```python
from build123d import *

# Parameters (mm, degrees)
SKETCH_1_R      = 1.55
SKETCH_1_R_2    = 14
EXTRUDE_1_DEPTH = 2


with BuildPart() as part:
    # 草图1 → 凸台-拉伸1 (new body)
    with BuildSketch(Plane.XY):
        Polygon((-90.5, 18), (-90.5, -18), (-62.5, -18), (-62.5, -46), (62.5, -46), (62.5, -18), (90.5, -18), (90.5, 18), (62.5, 18), (62.5, 46), (-62.5, 46), (-62.5, 18), align=None)
        with Locations((-52.935028843, -13.435028843)):
            Circle(SKETCH_1_R, mode=Mode.SUBTRACT)
        with Locations((-52.935028843, 13.435028843)):
            Circle(SKETCH_1_R, mode=Mode.SUBTRACT)
        with Locations((-26.064971157, -13.435028843)):
            Circle(SKETCH_1_R, mode=Mode.SUBTRACT)
        with Locations((-26.064971157, 13.435028843)):
            Circle(SKETCH_1_R, mode=Mode.SUBTRACT)
        with Locations((-39.5, 0)):
            Circle(SKETCH_1_R_2, mode=Mode.SUBTRACT)
        with Locations((39.5, 0)):
            Circle(SKETCH_1_R_2, mode=Mode.SUBTRACT)
        with Locations((57.5, -43)):
            Circle(SKETCH_1_R, mode=Mode.SUBTRACT)
        with Locations((37.5, -43)):
            Circle(SKETCH_1_R, mode=Mode.SUBTRACT)
        with Locations((-57.5, -43)):
            Circle(SKETCH_1_R, mode=Mode.SUBTRACT)
        with Locations((-37.5, -43)):
            Circle(SKETCH_1_R, mode=Mode.SUBTRACT)
        with Locations((-57.5, 43)):
            Circle(SKETCH_1_R, mode=Mode.SUBTRACT)
        with Locations((-37.5, 43)):
            Circle(SKETCH_1_R, mode=Mode.SUBTRACT)
        with Locations((37.5, 43)):
            Circle(SKETCH_1_R, mode=Mode.SUBTRACT)
        with Locations((57.5, 43)):
            Circle(SKETCH_1_R, mode=Mode.SUBTRACT)
        with Locations((15, -43)):
            Circle(SKETCH_1_R, mode=Mode.SUBTRACT)
        with Locations((-5, -43)):
            Circle(SKETCH_1_R, mode=Mode.SUBTRACT)
        with Locations((-5, 43)):
            Circle(SKETCH_1_R, mode=Mode.SUBTRACT)
        with Locations((15, 43)):
            Circle(SKETCH_1_R, mode=Mode.SUBTRACT)
        with Locations((-87.5, 8)):
            Circle(SKETCH_1_R, mode=Mode.SUBTRACT)
        with Locations((-87.5, -2)):
            Circle(SKETCH_1_R, mode=Mode.SUBTRACT)
        with Locations((87.5, 8)):
            Circle(SKETCH_1_R, mode=Mode.SUBTRACT)
        with Locations((87.5, -2)):
            Circle(SKETCH_1_R, mode=Mode.SUBTRACT)
        with Locations((26.064971157, 13.435028843)):
            Circle(SKETCH_1_R, mode=Mode.SUBTRACT)
        with Locations((52.935028843, 13.435028843)):
            Circle(SKETCH_1_R, mode=Mode.SUBTRACT)
        with Locations((52.935028843, -13.435028843)):
            Circle(SKETCH_1_R, mode=Mode.SUBTRACT)
        with Locations((26.064971157, -13.435028843)):
            Circle(SKETCH_1_R, mode=Mode.SUBTRACT)
        with BuildLine():
            Line((-81.106273476, 14), (-65, 14))
            ThreePointArc((-65, 14), (-64.646446609, 13.853553391), (-64.5, 13.5))
            Line((-64.5, 13.5), (-64.5, -10.235560912))
            ThreePointArc((-64.5, -10.235560912), (-64.853147938, -10.713509101), (-65.413737887, -10.516311621))
            Line((-65.413737887, -10.516311621), (-81.520011363, 13.219249291))
            ThreePointArc((-81.520011363, 13.219249291), (-81.548073971, 13.734120317), (-81.106273476, 14))
        make_face(mode=Mode.SUBTRACT)
        with BuildLine():
            Line((-66.893726524, -14), (-83, -14))
            ThreePointArc((-83, -14), (-83.353553391, -13.853553391), (-83.5, -13.5))
            Line((-83.5, -13.5), (-83.5, 10.235560912))
            ThreePointArc((-83.5, 10.235560912), (-83.146852062, 10.713509101), (-82.586262113, 10.516311621))
            Line((-82.586262113, 10.516311621), (-66.479988637, -13.219249291))
            ThreePointArc((-66.479988637, -13.219249291), (-66.451926029, -13.734120317), (-66.893726524, -14))
        make_face(mode=Mode.SUBTRACT)
        with BuildLine():
            Line((-45.012081811, 39), (-3, 39))
            ThreePointArc((-3, 39), (-2.292893219, 38.707106781), (-2, 38))
            Line((-2, 38), (-2, 32.601058551))
            ThreePointArc((-2, 32.601058551), (-2.3483514, 31.842537554), (-3.150708205, 31.61248026))
            Line((-3.150708205, 31.61248026), (-45.087435913, 38.005710855))
            ThreePointArc((-45.087435913, 38.005710855), (-45.510652053, 38.537785098), (-45.012081811, 39))
        make_face(mode=Mode.SUBTRACT)
        with BuildLine():
            Line((58.5, 38.5), (58.5, 22.795865962))
            ThreePointArc((58.5, 22.795865962), (58.3258243, 22.416605463), (57.924645897, 22.301576816))
            Line((57.924645897, 22.301576816), (2.849291795, 30.697783629))
            ThreePointArc((2.849291795, 30.697783629), (2.241479003, 31.03471332), (2, 31.686361919))
            Line((2, 31.686361919), (2, 38))
            ThreePointArc((2, 38), (2.292893219, 38.707106781), (3, 39))
            Line((3, 39), (58, 39))
            ThreePointArc((58, 39), (58.353553391, 38.853553391), (58.5, 38.5))
        make_face(mode=Mode.SUBTRACT)
        with BuildLine():
            Line((43.940148136, 21), (3, 21))
            ThreePointArc((3, 21), (2.292893219, 21.292893219), (2, 22))
            Line((2, 22), (2, 27.235525762))
            ThreePointArc((2, 27.235525762), (2.3483514, 27.994046759), (3.150708205, 28.224104053))
            Line((3.150708205, 28.224104053), (44.015502239, 21.994289145))
            ThreePointArc((44.015502239, 21.994289145), (44.438718378, 21.462214902), (43.940148136, 21))
        make_face(mode=Mode.SUBTRACT)
        with BuildLine():
            Line((-58.5, 21.5), (-58.5, 37.040718351))
            ThreePointArc((-58.5, 37.040718351), (-58.3258243, 37.41997885), (-57.924645897, 37.535007497))
            Line((-57.924645897, 37.535007497), (-2.849291795, 29.138800685))
            ThreePointArc((-2.849291795, 29.138800685), (-2.241479003, 28.801870993), (-2, 28.150222394))
            Line((-2, 28.150222394), (-2, 22))
            ThreePointArc((-2, 22), (-2.292893219, 21.292893219), (-3, 21))
            Line((-3, 21), (-58, 21))
            ThreePointArc((-58, 21), (-58.353553391, 21.146446609), (-58.5, 21.5))
        make_face(mode=Mode.SUBTRACT)
        with BuildLine():
            Line((-58, -21), (-3, -21))
            ThreePointArc((-3, -21), (-2.292893219, -21.292893219), (-2, -22))
            Line((-2, -22), (-2, -28.076121659))
            ThreePointArc((-2, -28.076121659), (-2.24106459, -28.72728757), (-2.848034087, -29.064507394))
            Line((-2.848034087, -29.064507394), (-57.924017044, -37.532529251))
            ThreePointArc((-57.924017044, -37.532529251), (-58.325582956, -37.417804089), (-58.5, -37.038336384))
            Line((-58.5, -37.038336384), (-58.5, -21.5))
            ThreePointArc((-58.5, -21.5), (-58.353553391, -21.146446609), (-58, -21))
        make_face(mode=Mode.SUBTRACT)
        with BuildLine():
            Line((57.5, -22.796852072), (57.5, -38.5))
            ThreePointArc((57.5, -38.5), (57.353553391, -38.853553391), (57, -39))
            Line((57, -39), (3, -39))
            ThreePointArc((3, -39), (2.292893219, -38.707106781), (2, -38))
            Line((2, -38), (2, -31.605315172))
            ThreePointArc((2, -31.605315172), (2.24106459, -30.954149261), (2.848034087, -30.616929437))
            Line((2.848034087, -30.616929437), (56.924017044, -22.302659205))
            ThreePointArc((56.924017044, -22.302659205), (57.325582956, -22.417384367), (57.5, -22.796852072))
        make_face(mode=Mode.SUBTRACT)
        Polygon((64.5, 14), (82.049806487, 14), (64.5, -11.862872718), align=None, mode=Mode.SUBTRACT)
        Polygon((83.5, 11.862872718), (83.5, -14), (65.950193513, -14), align=None, mode=Mode.SUBTRACT)
        with BuildLine():
            Line((-15.443413448, 17), (18, 17))
            ThreePointArc((18, 17), (18.353553391, 16.853553391), (18.5, 16.5))
            Line((18.5, 16.5), (18.5, -14.23178533))
            ThreePointArc((18.5, -14.23178533), (18.201051831, -14.689582405), (17.661687355, -14.599949091))
            Line((17.661687355, -14.599949091), (-15.781726092, 16.13183624))
            ThreePointArc((-15.781726092, 16.13183624), (-15.909289976, 16.681546302), (-15.443413448, 17))
        make_face(mode=Mode.SUBTRACT)
        with BuildLine():
            Line((15.443413448, -17), (-18, -17))
            ThreePointArc((-18, -17), (-18.353553391, -16.853553391), (-18.5, -16.5))
            Line((-18.5, -16.5), (-18.5, 14.23178533))
            ThreePointArc((-18.5, 14.23178533), (-18.201051831, 14.689582405), (-17.661687355, 14.599949091))
            Line((-17.661687355, 14.599949091), (15.781726092, -16.13183624))
            ThreePointArc((15.781726092, -16.13183624), (15.909289976, -16.681546302), (15.443413448, -17))
        make_face(mode=Mode.SUBTRACT)
        with BuildLine():
            Line((2, -22), (2, -27.153611911))
            ThreePointArc((2, -27.153611911), (2.348834089, -27.912547321), (3.151965913, -28.141997647))
            Line((3.151965913, -28.141997647), (43.137265542, -21.994192868))
            ThreePointArc((43.137265542, -21.994192868), (43.559828689, -21.461897728), (43.061282586, -21))
            Line((43.061282586, -21), (3, -21))
            ThreePointArc((3, -21), (2.292893219, -21.292893219), (2, -22))
        make_face(mode=Mode.SUBTRACT)
        with BuildLine():
            Line((-2, -38), (-2, -32.52782492))
            ThreePointArc((-2, -32.52782492), (-2.348834089, -31.76888951), (-3.151965913, -31.539439185))
            Line((-3.151965913, -31.539439185), (-45.209199217, -38.005807132))
            ThreePointArc((-45.209199217, -38.005807132), (-45.631762364, -38.538102272), (-45.133216261, -39))
            Line((-45.133216261, -39), (-3, -39))
            ThreePointArc((-3, -39), (-2.292893219, -38.707106781), (-2, -38))
        make_face(mode=Mode.SUBTRACT)
    extrude(amount=EXTRUDE_1_DEPTH)


solid = part.part
```
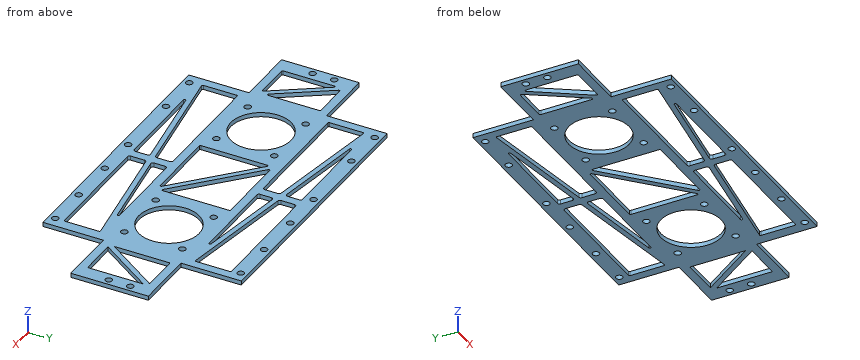
Check sheet for the modelled part. Datum: model origin and axes. Units: mm. Give positions to 0.01 mm unless a question says otherwise; leave off trailing zeros. Order: outer loops, then holes, each group sorted by start corner. A loop starts at its lowest first (then second) coordinate and runs counter-clockwise, first axis right, second up. Notation, with made-up numbers: (-12.75, -14) -> (28.25, -14) arc R28 cw to (28.25, 8) -> close; hole circle Ø8 at (74, 55.5). An arc over 180 degrees is marked (long way). Return JSON: item names as keys, results as strings.
1. Cross-section at B-B, the plane z = 1.7. Count the separate pieces of the cut face and the enclosed holes in it, plus the area to 3 significant figures.
From the geometry:
{"separate pieces": "1", "enclosed holes": "40", "area": "6,550 mm^2"}
2. Material ranges on probe 1 along Y at (x, z) = (-57.5, 1.2); probe 2 along Y at (x, z) = (-48, 1.35); probe 3 along Y at (x, z) = (-28, 1.8), recorded low to high. Write a range as [from, to].
From the geometry:
{"probe 1": "[-46, -44.55], [-41.45, -37.47], [-21, 21], [37.47, 41.45], [44.55, 46]", "probe 2": "[-46, -36.01], [-21, -11.12], [11.12, 21], [36.02, 46]", "probe 3": "[-46, -39], [-35.36, -32.93], [-21, -7.98], [7.98, 21], [32.97, 35.4], [39, 46]"}
3. Go/stop test with flat-tipped pins: P1, Ø0.6, axis at y = 33.5, z = 1, coming from the +X side; P2, Ø1.9, axis at x = 57.5, y = -43, coming from the -Z side; P3, Ø1, axis at x = -71, z = 1, coming from the -Y side; P4, Ø0.6, axis at y = 37, z = 1.5, coming from the -X side. Record where each tip stops, or that it passes through.
From the geometry:
{"P1": "x = 62.5", "P2": "through", "P3": "y = -18", "P4": "x = -62.5"}
4. Cross-section at A-A, the plane x = -41.5. Record the cut outline in (y, z).
From the geometry:
{"outline": "(-46, 0) -> (-39, 0) -> (-39, 2) -> (-46, 2) -> close; (-37.44, 0) -> (-35.01, 0) -> (-35.01, 2) -> (-37.44, 2) -> close; (-21, 0) -> (-13.86, 0) -> (-13.86, 2) -> (-21, 2) -> close; (13.86, 0) -> (21, 0) -> (21, 2) -> (13.86, 2) -> close; (35.03, 0) -> (37.46, 0) -> (37.46, 2) -> (35.03, 2) -> close; (39, 0) -> (46, 0) -> (46, 2) -> (39, 2) -> close"}
